Verification items for the finished model (mm, model axes). A direction names the side the tool comes from. Coordinates: 2 decimals unless noted, no trailing zeros. Loops run counter-clockwise (first coordinate to the right, second up) from the corner with the lowest first, then second, coordinate; pieces in that order, holes last. Notation, with made-up numbers: M 64.5,-38 L 116.5,-38 A17 cw 116.5,-13 Z; hole C 30.5,64 d4. An arc over 180 degrees is marked long. Write item = value, one per line. Start each with the question number.
```python
from build123d import *

# Parameters (mm, degrees)
FILLET_1_R = 2
FILLET_2_R = 2
FILLET_3_R = 2
FILLET_4_R = 2


with BuildPart() as part:
    # 草图1 → 旋转1 (revolve)
    with BuildSketch(Plane.XY):
        Polygon((0, 70.055695547), (0, -29.530111316), (-30.991998015, -29.530111316), (-30.991998015, 5.262792116), (-56.428826574, 5.262792116), (-56.428826574, 35.262792116), (-30.991998015, 35.262792116), (-30.991998015, 70.055695547), align=None)
        Polygon((0, 100.055695547), (0, 70.055695547), (-30.991998015, 70.055695547), align=None)
        Polygon((0, -29.530111316), (0, -59.530111316), (-30.991998015, -29.530111316), align=None)
    revolve(axis=Axis((0, 70.055695547, 0), (0, -1, 0)))

    # 圆角1
    fillet_1_edges = [part.edges().sort_by_distance(p)[0] for p in [
        (56.428826574, 35.262792116, 0),
    ]]
    fillet(fillet_1_edges, radius=FILLET_1_R)

    # 圆角2
    fillet_2_edges = [part.edges().sort_by_distance(p)[0] for p in [
        (56.428826574, 5.262792116, 0),
    ]]
    fillet(fillet_2_edges, radius=FILLET_2_R)

    # 圆角3
    fillet_3_edges = [part.edges().sort_by_distance(p)[0] for p in [
        (30.991998015, 70.055695547, 0),
    ]]
    fillet(fillet_3_edges, radius=FILLET_3_R)

    # 圆角4
    fillet_4_edges = [part.edges().sort_by_distance(p)[0] for p in [
        (30.991998015, -29.530111316, 0),
    ]]
    fillet(fillet_4_edges, radius=FILLET_4_R)


solid = part.part
```
Q1. Sectioned sample at B-B on y = 58. Record the cut outline in (x, z), plus the area to 3 significant figures.
Q2. Gauge pin test, flat ends, axial feed: pin 1 (2 mm diameter, centred on x = -4.5, z = 15, fed in from +Y); pin 2 (10 mm diameter, centred on y = 69.5, z = 38.5, fed in from -X); pin 3 (4 mm diameter, centred on x = 21.5, z = 8, fed in from -Y); pin 4 (4 mm diameter, centred on x = -28.5, y = 24, fed in from -Z). Record the tip position at first contact, or that the pin passes through.
Q3. Set-up check for faces 1 (the face through (23, 5.263, 23)), 2 (the face through (-14.301, 52.473, 27.495)), 3 (the face through (12.233, 20.445, 55.087)): record each of +Z, -Z, +X, -X, +Y, -Y from which the full face is reachable in a straight line by a thin tool's end or side.
Q4. Scan lines: L1, parallel to Y at x = -31, z = -8; L2, parallel to Z at x = 5, y = -37.5; L3, parallel to Z at x = 23, y = -2.5. Record each from-to range of solid material in increasing order. Write a range as [from, to].
Q5. Sectioned sample at A-A on y = 26.5. Record the cut outline in (x, z).
Solutions:
q1.outline = C 0,0 d61.98
q1.area = 3,020 mm²
q2.pin_1 = 85.86
q2.pin_2 = through
q2.pin_3 = -39.26
q2.pin_4 = -49.82
q3.face_1 = -Y
q3.face_2 = +Y
q3.face_3 = +Y, -Y
q4.L1 = [5.26, 35.26]
q4.L2 = [-22.2, 22.2]
q4.L3 = [-20.77, 20.77]
q5.outline = C 0,0 d112.86
